Read the model definition and answer for the solid it produces. Units are mm, in the model's axes. A direction names the side the tool comes from. Give positions to 0.01 mm unless a question says otherwise; leave off trailing zeros. Order: outer loops, then holes, each group sorted by start corner. A loop starts at its lowest first (then second) coordinate and runs counter-clockwise, first axis right, second up. Notation, with made-up numbers: (-6.5, 83) -> (31.5, 83) arc R14 cw to (31.5, 108) -> close; hole circle Ø7 at (59.5, 33). An arc over 180 degrees is marked (long way). One line per question, with ' | ' between items. Start each with the question number.
```python
from build123d import *

# Parameters (mm, degrees)
F0_R     = 63.5
F1_DEPTH = 45.72
F2_R     = 53.34
F3_DEPTH = 50.8
F4_R     = 58.42
F5_DEPTH = 45.72
F6_R     = 52.07
F7_DEPTH = 127


with BuildPart() as f1:
    # F0 (on Top) → F1 (new body)
    with BuildSketch(Plane.XY):
        Circle(F0_R)
    extrude(amount=F1_DEPTH)

    # F2 (on face) → F3 (cut)
    with BuildSketch(Plane.XY.offset(45.72)):
        Circle(F2_R)
    extrude(amount=-F3_DEPTH, mode=Mode.SUBTRACT)

    # F4 (on Top) → F5 (join)
    with BuildSketch(Plane.XY):
        Circle(F4_R)
    extrude(amount=-F5_DEPTH)

    # F6 (on face) → F7 (cut)
    with BuildSketch(Plane(origin=(0, 0, -45.72), x_dir=(1, 0, 0), z_dir=(0, 0, -1))):
        Circle(F6_R)
    extrude(amount=-F7_DEPTH, mode=Mode.SUBTRACT)


solid = f1.part
```
Q1. A cutting plane is placed at C-C, the plane z = 5. Determine the outline of the cut face in (x, y).
Q2. Determine the mould class of faces 3 (the flat face through (12, -51, 0)), 4 (the cylindrical face through (-13.77, -61.99, 22.54)), 5 (the cylindrical face through (-6.944, 52.886, 23.18)), 6 (the flat face through (-52.2, -4.1, -45.72)) for opening direction Y: pulls with the +Y half, pulls with the -Y half, needs draft (parallel to the pull), parting line crosses it, or undercut.
Q3. Given P1, Ø10, axis at x = -50.5, y = 41, coming from the +Z side; P2, Ø12, axis at x = -34.5, z = -30.5, coming from the -Y side; P3, Ø4, axis at x = -9, y = 49.5, coming from the +Z side; P4, Ø2, axis at y = 20, z = -1.5, coming from the +X side, each flat-ended and moving along its own axis, determine where each tip first touches the part or whether it passes through.
Q4. A cutting plane is placed at D-D, the plane x = 56. Determine the outline of the cut face in (y, z).
Q5. Which of the six approach directions +Z, -Z, +X, -X, +Y, -Y give full straight-line access (tool end or side, diameter ignored) to faces 1 (the cylindrical face through (-43.06, 39.48, -22.54)), 2 (the flat face through (-14, 52, 45.72))?
Q6. Find the intervals of material crossed by line 1 (Y direction, x = 0, z = 11.5); line 2 (Y direction, x = 0, z = -14); line 3 (Z direction, x = -38, y = 48.5), in increasing order.
Q7. A cutting plane is placed at A-A, the plane y = 0. Determine the outline of the cut face in (x, z).
Geometry results:
1) outline: circle Ø127 at (0, 0); hole circle Ø106.68 at (0, 0)
2) face 3: undercut | face 4: parting line crosses it | face 5: undercut | face 6: needs draft
3) P1: z = 45.72 | P2: y = -51 | P3: z = 0 | P4: x = 55.24
4) outline: (-29.94, 0) -> (-16.64, 0) -> (-16.64, -45.72) -> (16.64, -45.72) -> (16.64, 0) -> (29.94, 0) -> (29.94, 45.72) -> (-29.94, 45.72) -> close
5) face 1: -Z | face 2: +Z, +X, -X, +Y, -Y
6) line 1: -63.5 to -53.34, 53.34 to 63.5 | line 2: -58.42 to -52.07, 52.07 to 58.42 | line 3: 0 to 45.72
7) outline: (-63.5, 0) -> (-58.42, 0) -> (-58.42, -45.72) -> (-52.07, -45.72) -> (-52.07, 0) -> (-53.34, 0) -> (-53.34, 45.72) -> (-63.5, 45.72) -> close; (52.07, -45.72) -> (58.42, -45.72) -> (58.42, 0) -> (63.5, 0) -> (63.5, 45.72) -> (53.34, 45.72) -> (53.34, 0) -> (52.07, 0) -> close
